```python
from build123d import *

# Parameters (mm, degrees)
CYLINDER_R     = 10
CYLINDER_DEPTH = 10
THICKNESS_T    = 2


with BuildPart() as cilindro:
    # Cylinder → Cylinder (new body)
    with BuildSketch(Plane.XY.offset(-5)):
        Circle(CYLINDER_R)
    extrude(amount=CYLINDER_DEPTH)


with BuildPart() as cut:
    # Cone → Cone (revolve)
    with BuildSketch(Plane.XZ):
        Polygon((0, 0), (40, 0), (60, 100), (0, 100), align=None)
    revolve(axis=Axis((0, 0, 0), (0, 0, 1)))

    # Thickness
    thickness_openings = [cut.faces().sort_by_distance(p)[0] for p in [
        (0, 0, 100),
    ]]
    offset(amount=THICKNESS_T, openings=thickness_openings, kind=Kind.INTERSECTION)

    # Cut: cut Cilindro
    add(cilindro.part, mode=Mode.SUBTRACT)


solid = cut.part
```
Input: part model. Units: mm. Frame: model coordinates. A direction names the side the tool comes from. Coordinates: 2 decimals unless noted, no trailing zeros. Order: outer loops, then holes, each group sorted by start corner. A loop starts at its lowest first (then second) coordinate and runs counter-clockwise, first axis right, second up. Notation, with made-up numbers: (23, 63) - (74, 63) arc R16 cw to (74, 91) - close; hole circle Ø1 at (-7.5, -13). An arc over 180 degrees is marked (long way). Return JSON: item names as keys, results as strings.
Q1. Cut plane A-A (y = 0). Return loops of the section in (x, z).
The answers:
{"outline": "(-62.04, 100) - (-41.64, -2) - (-10, -2) - (-10, 0) - (-40, 0) - (-60, 100) - close; (10, -2) - (41.64, -2) - (62.04, 100) - (60, 100) - (40, 0) - (10, 0) - close"}
Q2. First-contact query: pin 1 (8 mm diameter, centred on x = 27, z = 33.5, fed in from -Y); pin 2 (4 mm diameter, centred on y = -33.5, z = 55.5, fed in from +X); pin 3 (10 mm diameter, centred on y = -33.5, z = 63.5, fed in from -X). Flat tips, straight axial feed; report the tip coordinate or a pass-through.
The answers:
{"pin 1": "stops at y = -43.16", "pin 2": "stops at x = 42.88", "pin 3": "stops at x = -46.95"}
Q3. Draft query along Y for faces 3 (the conical face through (44.264, -18.353, 39.589)), 4 (the flat face through (-32, 51, 100)), 5 (the conical face through (-10.777, -48.534, 38.381)). Return one class per face: +Y half, -Y half, draft (parallel to the pull), parting line (faces both ways), or undercut.
The answers:
{"face 3": "undercut", "face 4": "draft", "face 5": "parting line"}
Q4. Access query for faces 1 (the flat face through (-8, -8, 0)), 2 (the flat face through (-9, -9, -2)). Directions: +Z, -Z, +X, -X, +Y, -Y. A direction counts if a zero-diameter tool reaches every point of the face in a straight line with its end or side. Return the directions, or none.
The answers:
{"face 1": "+Z", "face 2": "-Z, +X, -X, +Y, -Y"}
Q5. Cut plane D-D (z = 12). Return loops of the section in (x, y), then the cut area to 3 significant figures.
The answers:
{"outline": "circle Ø88.88 at (0, 0); hole circle Ø84.8 at (0, 0)", "area": "556 mm2"}
Q6. Cut plane C-C (z = 61). Return loops of the section in (x, y), then the cut area to 3 significant figures.
The answers:
{"outline": "circle Ø108.48 at (0, 0); hole circle Ø104.4 at (0, 0)", "area": "682 mm2"}
Q7. Ray query, probe 1 along Z at (x, y) = (-9, -29.5); probe 2 along X at (y, z) = (37.5, 11); probe 3 along X at (y, z) = (0, -0.75). Return the intervals inside material, ascending.
The answers:
{"probe 1": "z = -2 to 0", "probe 2": "x = -23.47 to -19.35, 19.35 to 23.47", "probe 3": "x = -41.89 to -10, 10 to 41.89"}
